Here's the drawing with two shaded views (mm, measured from the low corner). I have some questions. A direction names the side the tool comes from. Round coordinates to 2 decimals unless told otherwise and drop trailing zeros. Order: outer loops, then holes, each group sorted by start corner. A loop starts at its lowest first (then second) coordinate and runs counter-clockwise, first axis right, second up.
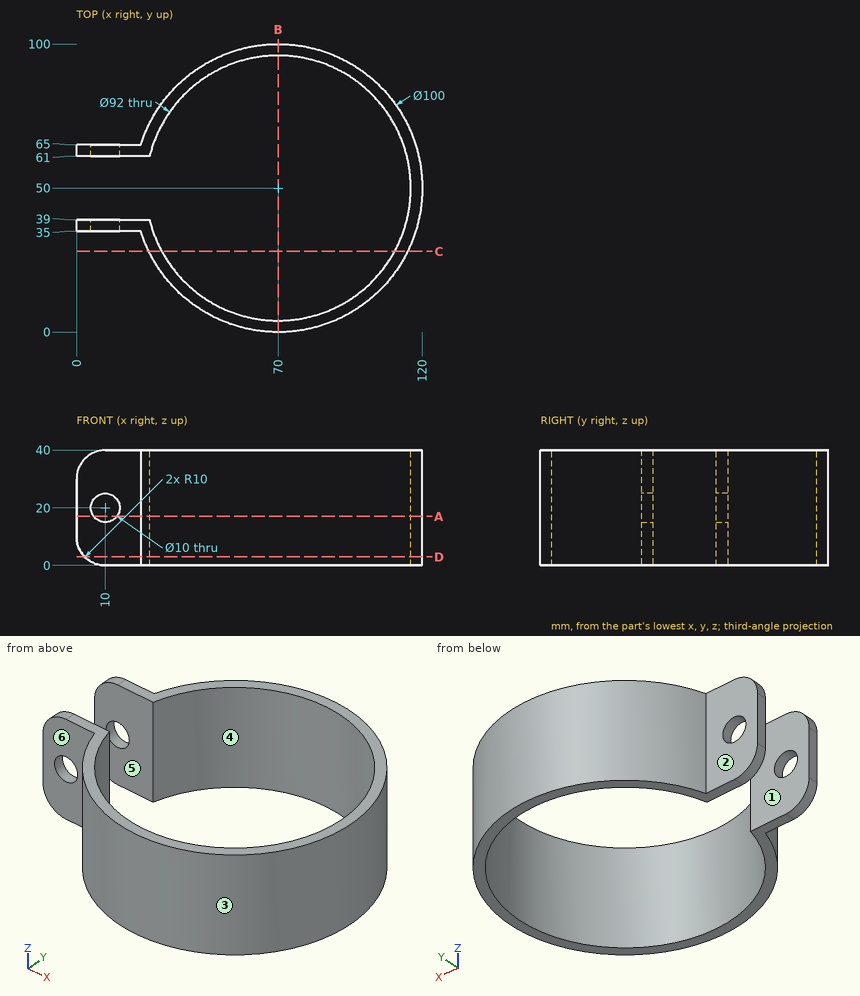
Q1. For the marked faces 4, 5 and 6, which set-ups out of +Z, -Z, +X, -X, +Y, -Y let a thin tool reach every point of the face, with its end or its side?
Q2. Imagine slicing it at A-A, the plane z = 17. Please give me the cut outline in (x, y).
Q3. Imagine slicing it at D-D, the plane z = 3. Please give me the cut outline in (x, y).
Q4. We'd pull the mould along Y, two halves only. Please class the marked faces 1, 2 and 3: released by +Y, released by -Y, zero draft, split by the parting line, or undercut.
Q5. I need wall thicknesses on L1, parallel to Y at x = 70, z = 27; L2, parallel to X at y = 63.7, z = 20; L3, parallel to X at y = 63.15, z = 20. Which ranges of each line are inside material? Lowest first, please.
Q6. Imagine slicing it at B-B, the plane x = 70. Please give me the cut outline in (y, z).
Q7. For P1, Ø3, axis at y = 42.5, z = 14.5, coming from the -X side; P2, Ø18, axis at x = 9, z = 20, coming from the +Y side; P3, Ø1, axis at y = 53, z = 20.5, coming from the +X side, each with a flat end and sliding along its axis, tell me the tip position at first contact or that it passes through.
Q8. Imagine slicing it at C-C, the plane y = 28. Please give me the cut outline in (x, z), then the cut area to 3 significant figures.
Filled in:
1. face 4: +Z, -Z
1. face 5: +Z, -Z, -X
1. face 6: +Z, -Z, -X, -Y
2. outline: (0, 35) - (6, 35) - (6, 39) - (0, 39) - close; (0, 61) - (6, 61) - (6, 65) - (0, 65) - close; (14, 35) - (22.3, 35) arc R50 ccw (long way) to (22.3, 65) - (14, 65) - (14, 61) - (25.33, 61) arc R46 cw (long way) to (25.33, 39) - (14, 39) - close
3. outline: (2.86, 35) - (22.3, 35) arc R50 ccw (long way) to (22.3, 65) - (2.86, 65) - (2.86, 61) - (25.33, 61) arc R46 cw (long way) to (25.33, 39) - (2.86, 39) - close
4. face 1: undercut
4. face 2: released by +Y
4. face 3: split by the parting line
5. L1: y = 0 to 4, 96 to 100
5. L2: x = 0 to 5, 15 to 26.09, 113.91 to 118.09
5. L3: x = 0 to 5, 15 to 25.92, 114.08 to 118.24
6. outline: (0, 0) - (4, 0) - (4, 40) - (0, 40) - close; (96, 0) - (100, 0) - (100, 40) - (96, 40) - close
7. P1: stops at x = 115.11
7. P2: stops at y = 65
7. P3: stops at x = 119.94
8. outline: (25.1, 0) - (29.6, 0) - (29.6, 40) - (25.1, 40) - close; (110.4, 0) - (114.9, 0) - (114.9, 40) - (110.4, 40) - close
8. area: 360 mm2
